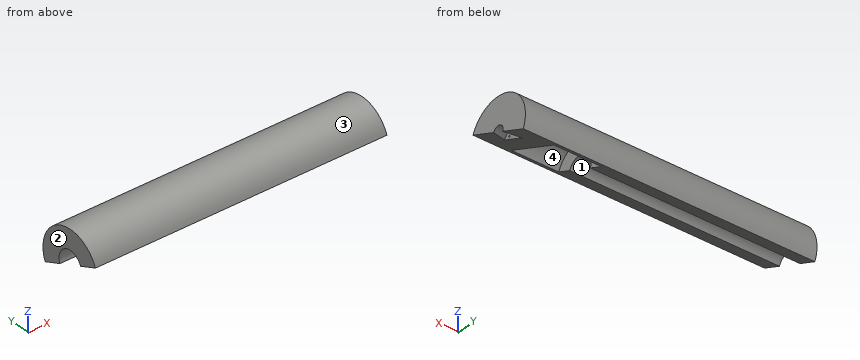
from build123d import *

# Parameters (mm, degrees)
CUT_EXTRUDE1_REACH = 247.25
SKETCH3_R          = 0.80645
SKETCH4_W          = 62
SKETCH4_H          = 273.6661
CUT_EXTRUDE2_DEPTH = 278.155433447


with BuildPart() as part:
    # Sketch1 → Revolve1 (revolve)
    with BuildSketch(Plane.XY, mode=Mode.PRIVATE) as revolve1_sk:
        Polygon((0, 12.7), (196.85, 12.7), (196.85, 26.162), (241.3, 26.162), (241.3, 0), (259.36, 0), (259.36, 10.7696), (273.6661, 5.5626), (273.6661, 31), (0, 31), align=None)
    revolve(revolve1_sk.sketch.rotate(Axis((0, 0, 0), (1, 0, 0)), 90), axis=Axis((0, 0, 0), (1, 0, 0)))

    # Sketch3 → Cut-Extrude1 (cut, up to next)
    with BuildSketch(Plane.ZY.offset(-241.3), mode=Mode.PRIVATE) as cut_extrude1_sk1:
        with Locations((0, 6.477)):
            Circle(SKETCH3_R)
    cut_extrude1_tool1 = extrude(cut_extrude1_sk1.sketch, amount=-CUT_EXTRUDE1_REACH, mode=Mode.PRIVATE) & part.part
    # Sketch3 → Cut-Extrude1 (cut, up to next)
    with BuildSketch(Plane.ZY.offset(-241.3), mode=Mode.PRIVATE) as cut_extrude1_sk2:
        with Locations((4.579930622, 4.579930622)):
            Circle(SKETCH3_R)
    cut_extrude1_tool2 = extrude(cut_extrude1_sk2.sketch, amount=-CUT_EXTRUDE1_REACH, mode=Mode.PRIVATE) & part.part
    # Sketch3 → Cut-Extrude1 (cut, up to next)
    with BuildSketch(Plane.ZY.offset(-241.3), mode=Mode.PRIVATE) as cut_extrude1_sk3:
        with Locations((6.477, 0)):
            Circle(SKETCH3_R)
    cut_extrude1_tool3 = extrude(cut_extrude1_sk3.sketch, amount=-CUT_EXTRUDE1_REACH, mode=Mode.PRIVATE) & part.part
    # Sketch3 → Cut-Extrude1 (cut, up to next)
    with BuildSketch(Plane.ZY.offset(-241.3), mode=Mode.PRIVATE) as cut_extrude1_sk4:
        with Locations((4.579930622, -4.579930622)):
            Circle(SKETCH3_R)
    cut_extrude1_tool4 = extrude(cut_extrude1_sk4.sketch, amount=-CUT_EXTRUDE1_REACH, mode=Mode.PRIVATE) & part.part
    # Sketch3 → Cut-Extrude1 (cut, up to next)
    with BuildSketch(Plane.ZY.offset(-241.3), mode=Mode.PRIVATE) as cut_extrude1_sk5:
        with Locations((0, -6.477)):
            Circle(SKETCH3_R)
    cut_extrude1_tool5 = extrude(cut_extrude1_sk5.sketch, amount=-CUT_EXTRUDE1_REACH, mode=Mode.PRIVATE) & part.part
    # Sketch3 → Cut-Extrude1 (cut, up to next)
    with BuildSketch(Plane.ZY.offset(-241.3), mode=Mode.PRIVATE) as cut_extrude1_sk6:
        with Locations((-4.579930622, -4.579930622)):
            Circle(SKETCH3_R)
    cut_extrude1_tool6 = extrude(cut_extrude1_sk6.sketch, amount=-CUT_EXTRUDE1_REACH, mode=Mode.PRIVATE) & part.part
    # Sketch3 → Cut-Extrude1 (cut, up to next)
    with BuildSketch(Plane.ZY.offset(-241.3), mode=Mode.PRIVATE) as cut_extrude1_sk7:
        with Locations((-6.477, 0)):
            Circle(SKETCH3_R)
    cut_extrude1_tool7 = extrude(cut_extrude1_sk7.sketch, amount=-CUT_EXTRUDE1_REACH, mode=Mode.PRIVATE) & part.part
    # Sketch3 → Cut-Extrude1 (cut, up to next)
    with BuildSketch(Plane.ZY.offset(-241.3), mode=Mode.PRIVATE) as cut_extrude1_sk8:
        with Locations((-4.579930622, 4.579930622)):
            Circle(SKETCH3_R)
    cut_extrude1_tool8 = extrude(cut_extrude1_sk8.sketch, amount=-CUT_EXTRUDE1_REACH, mode=Mode.PRIVATE) & part.part
    add(cut_extrude1_tool1.solids().sort_by_distance((241.3, 6.477, 0))[0], mode=Mode.SUBTRACT)
    add(cut_extrude1_tool2.solids().sort_by_distance((241.3, 4.579931, 4.579931))[0], mode=Mode.SUBTRACT)
    add(cut_extrude1_tool3.solids().sort_by_distance((241.3, 0, 6.477))[0], mode=Mode.SUBTRACT)
    add(cut_extrude1_tool4.solids().sort_by_distance((241.3, -4.579931, 4.579931))[0], mode=Mode.SUBTRACT)
    add(cut_extrude1_tool5.solids().sort_by_distance((241.3, -6.477, 0))[0], mode=Mode.SUBTRACT)
    add(cut_extrude1_tool6.solids().sort_by_distance((241.3, -4.579931, -4.579931))[0], mode=Mode.SUBTRACT)
    add(cut_extrude1_tool7.solids().sort_by_distance((241.3, 0, -6.477))[0], mode=Mode.SUBTRACT)
    add(cut_extrude1_tool8.solids().sort_by_distance((241.3, 4.579931, -4.579931))[0], mode=Mode.SUBTRACT)

    # Sketch4 → Cut-Extrude2 (cut, through all)
    with BuildSketch(Plane(origin=(0, 0, 0), x_dir=(0, -0.9238795325112865, 0.38268343236509056), z_dir=(0, 0.3826834323650905, 0.9238795325112864))):
        with Locations((0, 136.83305)):
            Rectangle(SKETCH4_W, SKETCH4_H)
    extrude(amount=-CUT_EXTRUDE2_DEPTH, mode=Mode.SUBTRACT)


solid = part.part
Check sheet for the modelled part. Datum: model origin and axes. Units: mm. Face numbers are marked on the shaded views. Round coordinates to 2 decimals unless told otherwise and drop trailing zeros. Loops run counter-clockwise (first coordinate to the right, second up) from the corner with the lowest first, then second, coordinate; pieces in that order, holes last.
1. Sectioned sample at B-B on y = -21. Record the boundary of the cut face in (x, z), and give its area (3 significant figures).
2. Scan lines: probe 1 along X at (y, z) = (8, 23); probe 2 along Y at (x, z) = (249, 0); probe 3 along Y at (x, z) = (145, 10.5). Record each from-to range of solid material in increasing order.
3. Sectioned sample at A-A on z = 17.5. Record the boundary of the cut face in (x, y), and give its area (3 significant figures).
4. Gauge pin test, flat ends, axial feed: pin 1 Ø8 at (y, z) = (-9, -0.5) entering from -X; pin 2 Ø1 at (x, z) = (178, 15) entering from -Y; pin 3 Ø3 at (x, z) = (53.5, 17.5) entering from -Y. Record the tip position at first contact, or that the pin passes through.
5. Mould release check, pull along Y, two halves, no side actions. Record for the marked faces 1, 2, 3 and 4: released by +Y, released by -Y, zero draft, split by the parting line, or undercut.
6. Sectioned sample at D-D on y = 21. Record the boundary of the cut face in (x, z), and give its area (3 significant figures).
Recorded:
1. outline: (0, 8.7) - (196.85, 8.7) - (196.85, 15.6) - (241.3, 15.6) - (241.3, 8.7) - (273.67, 8.7) - (273.67, 22.8) - (0, 22.8) - close
1. area: 3,550 mm2
2. probe 1: x = 0 to 196.85, 241.3 to 273.67
2. probe 2: y = 0 to 5.67, 7.28 to 31
2. probe 3: y = -25.35 to -7.14, 7.14 to 29.17
3. outline: (0, -25.59) - (273.67, -25.59) - (273.67, 25.59) - (0, 25.59) - close; hole (196.85, -19.45) - (241.3, -19.45) - (241.3, 19.45) - (196.85, 19.45) - close
3. area: 12,300 mm2
4. pin 1: stops at x = 241.3
4. pin 2: stops at y = -27.4
4. pin 3: stops at y = -26.55
5. face 1: undercut
5. face 2: zero draft
5. face 3: split by the parting line
5. face 4: undercut
6. outline: (0, -8.7) - (196.85, -8.7) - (196.85, 15.6) - (241.3, 15.6) - (241.3, -8.7) - (273.67, -8.7) - (273.67, 22.8) - (0, 22.8) - close
6. area: 7,540 mm2
